```python
from build123d import *

# Parameters (mm, degrees)
F0_R     = 1.15
F1_DEPTH = 4
F2_R     = 1.5
F3_DEPTH = 5
F4_R     = 1.5


with BuildPart() as f1:
    # F0 (on Front) → F1 (new body)
    with BuildSketch(Plane.XZ):
        with BuildLine():
            Line((-3.5, -3.1), (5, -3.1))
            Line((5, -3.1), (5, 3.1))
            Line((5, 3.1), (-3.5, 3.1))
            ThreePointArc((-3.5, 3.1), (-3.93934, 2.03934), (-5, 1.6))
            Line((-5, 1.6), (-5, -1.6))
            ThreePointArc((-5, -1.6), (-3.93934, -2.03934), (-3.5, -3.1))
        make_face()
        with Locations((2.7, 0)):
            Circle(F0_R, mode=Mode.SUBTRACT)
    extrude(amount=F1_DEPTH)

    # F2 (on face) → F3 (cut)
    with BuildSketch(Plane(origin=(-5, 0, 0), x_dir=(0, -1, 0), z_dir=(-1, 0, 0))):
        with Locations((2, 0)):
            Circle(F2_R)
    extrude(amount=-F3_DEPTH, mode=Mode.SUBTRACT)

    # F4
    f4_edges = [f1.edges().sort_by_distance(p)[0] for p in [
        (0.75, -4, -3.1),
        (0.75, -4, 3.1),
        (0.75, 0, -3.1),
        (0.75, 0, 3.1),
    ]]
    fillet(f4_edges, radius=F4_R)


solid = f1.part
```
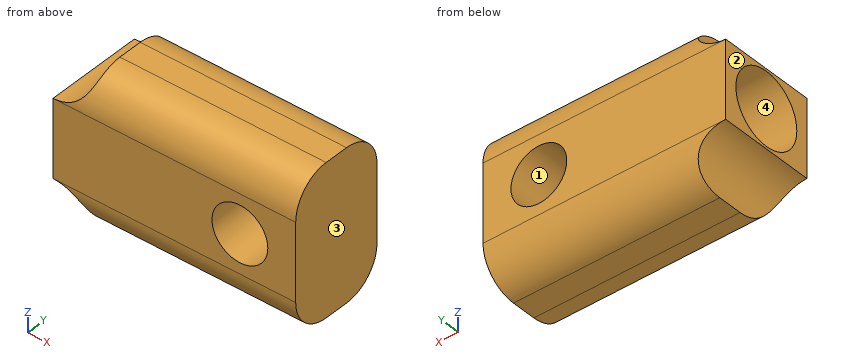
The listing builds one solid part. Answer for the finished solid, in the listing's coordinates (mm). Face numbers are marked on the shaded views. Coordinates: 2 decimals unless noted, no trailing zeros. Write each loop counter-clockwise with the first axis right and the second up, starting at its lowest first coordinate (ties: lowest second). Pieces come first, ordered by that corner, then holes. Notation, with made-up numbers: M 43,25 L 75,25 A30 cw 75,58 Z; hole C -19,32 d8. An arc over 180 degrees is marked long. Use a Markdown table: item, result. Add a question column.
1. Section D-D (y = -2) is taken. Give the vertices of the cut face in (x, z), plus the area to 3 significant figures.
2. Straight lines are drawn through the part: line 1 along Z through (x, y) = (2.75, -2); line 2 along Z through (x, y) = (-2.2, -2); line 3 along X through (y, z) = (-1.8, 0.25). For each, find the intervals that lie inside material, in ascending order. Write a range as [from, to].
3. Section C-C (x = -3) is taken. Give the vertices of the cut face in (y, z).
4. Section A-A (x = 2.7) is taken. Give the vertices of the cut face in (y, z).
5. Given P1, Ø1.8, axis at y = -2, z = 0, coming from the -X side, flat-ended and moving along its own axis, determine where the tip first touches the part or whether it passes through.
6. Section B-B (z = 0) is taken. Give the vertices of the cut face in (x, y), plus the area to 3 significant figures.
7. For a pull along X with two mould halves and no side action, classify the marked faces 1, 2, 3 and 4 as +X half, -X half, draft (parallel to the pull), parting line (faces both ways), or undercut.
Data:
| question | item | result |
|---|---|---|
| 1 | outline | M -5,-1.6 A1.5 cw -3.5,-3.1 L 5,-3.1 L 5,3.1 L -3.5,3.1 A1.5 cw -5,1.6 L -5,1.5 L 0,1.5 L 0,-1.5 L -5,-1.5 Z; hole C 2.7,0 d2.3 |
| 1 | area | 39.3 mm2 |
| 2 | line 1 | z = [-3.1, -1.15], [1.15, 3.1] |
| 2 | line 2 | z = [-3.1, -1.5], [1.5, 3.1] |
| 2 | line 3 | x = [0, 1.58], [3.82, 5] |
| 3 | outline | M -4,-1.6 A1.5 ccw -2.5,-3.1 L -1.5,-3.1 A1.5 ccw 0,-1.6 L 0,1.6 A1.5 ccw -1.5,3.1 L -2.5,3.1 A1.5 ccw -4,1.6 Z; hole C -2,0 d3 |
| 4 | outline | M -4,-1.6 A1.5 ccw -2.5,-3.1 L -1.5,-3.1 A1.5 ccw 0,-1.6 L 0,-1.15 L -4,-1.15 Z; M -4,1.15 L 0,1.15 L 0,1.6 A1.5 ccw -1.5,3.1 L -2.5,3.1 A1.5 ccw -4,1.6 Z |
| 5 | P1 | stops at x = 0 |
| 6 | outline | M -5,-4 L 1.55,-4 L 1.55,0 L -5,0 L -5,-0.5 L 0,-0.5 L 0,-3.5 L -5,-3.5 Z; M 3.85,-4 L 5,-4 L 5,0 L 3.85,0 Z |
| 6 | area | 15.8 mm2 |
| 7 | face 1 | undercut |
| 7 | face 2 | -X half |
| 7 | face 3 | +X half |
| 7 | face 4 | draft |
